The listing builds one solid part. Answer for the finished solid, in the listing's coordinates (mm). A direction names the side the tool comes from. Give positions to 0.01 mm unless a question says otherwise; leave off trailing zeros. Write each loop counter-clockwise with the first axis right and the second up, starting at its lowest first coordinate (ties: lowest second). Pieces come first, ordered by that corner, then holes. Notation, with made-up numbers: (44, -25.5) - (86, -25.5) arc R18 ccw to (86, 2.5) - close; hole circle Ø6 at (-17, 77). An arc over 180 degrees is marked (long way). Answer in a Markdown table with one row per item. Add a question column.
from build123d import *

# Parameters (mm, degrees)
F1_DEPTH = 3.175
F2_R     = 1.27
F3_R     = 0.508


with BuildPart() as f1:
    # F0 (on Top) → F1 (new body, symmetric)
    with BuildSketch(Plane.XY):
        Polygon((-6.35, 16.042595), (-6.35, 3.342595), (6.35, 3.342595), (6.35, 16.042595), (1.190625, 16.042595), (0.79375, 11.280095), (-0.79375, 11.280095), (-1.190625, 16.042595), align=None)
    extrude(amount=F1_DEPTH, both=True)

    # F2
    f2_edges = [f1.edges().sort_by_distance(p)[0] for p in [
        (-6.35, 3.342595, 0),
        (6.35, 3.342595, 0),
        (6.35, 16.042595, 0),
        (-6.35, 16.042595, 0),
    ]]
    fillet(f2_edges, radius=F2_R)

    # F3
    f3_edges = [f1.edges().sort_by_distance(p)[0] for p in [
        (1.190625, 16.042595, 0),
        (-1.190625, 16.042595, 0),
    ]]
    fillet(f3_edges, radius=F3_R)


solid = f1.part
1. Straight lines are drawn through the part: L1, parallel to Y at x = 0.75, z = -2.25; L2, parallel to X at y = 12.25, z = 0.25; L3, parallel to X at y = 14.25, z = -2.5. For each, find the intervals that lie inside material, in ascending order. Write a range as [from, to].
2. Given pin 1 Ø1.3 at (x, z) = (0, 0.5) entering from +Y, flat-ended and moving along its own axis, determine where the tip first touches the part or whether it passes through.
3. Section B-B (x = 0.25) is taken. Give the vertices of the cut face in (y, z) (3 decimals).
4. Section A-A (z = -2) is taken. Give the vertices of the cut face in (x, y), and give its area (3 significant figures).
5. A tool of negligible diameter and unlimited length cuts with its end or side. For faces 1 (the face through (0, 10, -3.175)), 2 (the face through (-0.97, 13.4, 0.04)), from which of +Z, -Z, +X, -X, +Y, -Y can it reach the whole face along a straight path? Write none if from no direction.
6. The mould has two halves that part along X. Classify faces 3 (the face through (-5.988, 3.724, 0.044)), 4 (the face through (3, 16.043, 0)), 5 (the face through (0, 11.28, 0)), 6 (the face through (0.975, 13.459, 0.044)): +X half, -X half, draft (parallel to the pull), parting line (faces both ways), or undercut.
Geometry check:
| question | item | result |
|---|---|---|
| 1 | L1 | [3.34, 11.28] |
| 1 | L2 | [-6.35, -0.87], [0.87, 6.35] |
| 1 | L3 | [-6.35, -1.04], [1.04, 6.35] |
| 2 | pin 1 | y = 11.28 |
| 3 | outline | (3.343, -3.175) - (11.28, -3.175) - (11.28, 3.175) - (3.343, 3.175) - close |
| 4 | outline | (-6.35, 4.61) arc R1.27 ccw to (-5.08, 3.34) - (5.08, 3.34) arc R1.27 ccw to (6.35, 4.61) - (6.35, 14.77) arc R1.27 ccw to (5.08, 16.04) - (1.66, 16.04) arc R0.51 ccw to (1.15, 15.58) - (0.79, 11.28) - (-0.79, 11.28) - (-1.15, 15.58) arc R0.51 ccw to (-1.66, 16.04) - (-5.08, 16.04) arc R1.27 ccw to (-6.35, 14.77) - close |
| 4 | area | 150 mm² |
| 5 | face 1 | -Z, +X, -X, +Y, -Y |
| 5 | face 2 | +Z, -Z, +Y |
| 6 | face 3 | -X half |
| 6 | face 4 | draft |
| 6 | face 5 | undercut |
| 6 | face 6 | undercut |
